Could you check a few things on this model? Use its own coordinates, in mm. A direction names the side the tool comes from. Coordinates: 2 decimals unless noted, no trailing zeros. Write each loop counter-clockwise with the first axis right and the second up, starting at its lowest first coordinate (ties: lowest second). Pieces come first, ordered by that corner, then holes.
```python
from build123d import *

# Parameters (mm, degrees)
BOSS_EXTRUDE1_DEPTH = 247.65
SKETCH2_R           = 2.286
CUT_EXTRUDE1_DEPTH  = 255.69929163
SKETCH3_R           = 2.286
CUT_EXTRUDE2_DEPTH  = 255.408366321
FILLET1_R           = 6.35


with BuildPart() as part:
    # Sketch1 → Boss-Extrude1 (new body)
    with BuildSketch(Plane.XY):
        Polygon((0, 0), (31.018857102, 0), (57.870573741, -9.773225596), (58.413530719, -8.28146356), (31.298776184, 1.5875), (0, 1.5875), align=None)
    extrude(amount=BOSS_EXTRUDE1_DEPTH)

    # Sketch2 → Cut-Extrude1 (cut, through all)
    with BuildSketch(Plane(origin=(0, 1.5875, 0), x_dir=(1, 0, 0), z_dir=(0, 1, 0))):
        with Locations(Location((4.7625, -6.35, 0), (0, 0, 180))):
            Circle(SKETCH2_R)
        with Locations(Location((4.7625, -241.3, 0), (0, 0, 180))):
            Circle(SKETCH2_R)
        with Locations(Location((4.7625, -82.55, 0), (0, 0, 180))):
            Circle(SKETCH2_R)
        with Locations(Location((4.7625, -165.1, 0), (0, 0, 180))):
            Circle(SKETCH2_R)
    extrude(amount=-CUT_EXTRUDE1_DEPTH, mode=Mode.SUBTRACT)

    # Sketch3 → Cut-Extrude2 (cut, through all)
    with BuildSketch(Plane(origin=(4.171473971, 11.461030541, 0), x_dir=(0.9396926207859064, -0.34202014332567426, 0), z_dir=(0.34202014332567426, 0.9396926207859064, 0))):
        with Locations(Location((45.023191124, -6.35, 0), (0, 0, 180))):
            Circle(SKETCH3_R)
        with Locations(Location((45.023191124, -241.3, 0), (0, 0, 180))):
            Circle(SKETCH3_R)
    extrude(amount=-CUT_EXTRUDE2_DEPTH, mode=Mode.SUBTRACT)

    # Fillet1
    fillet1_edges = [part.edges().sort_by_distance(p)[0] for p in [
        (58.14205223, -9.027344578, 0),
        (58.14205223, -9.027344578, 247.65),
    ]]
    fillet(fillet1_edges, radius=FILLET1_R)


solid = part.part
```
Item 1: I want a section at A-A, the plane z = 82.55. List the corners of the cut face in (x, y) for me, then the cut area to 3 significant figures.
Item 2: Which directions (+Z, -Z, +X, -X, +Y, -Y) give clear straight access to the entire face, cutting with the end or side of a thin tool? Please do faces 1 (the flat face through (26, 1, 247.65)), 2 (the flat face through (15, 0, 122)).
Item 3: I want a section at B-B, the plane x = 10. List the corners of the cut face in (y, z) for me.
Item 4: If I drill on line 1 along Z through (x, y) = (45, -5); line 2 along Y through (x, z) = (26, 226); line 3 along Y through (x, z) = (32, 50.5), over which ranges is the centre line in solid material (lowest first)?
Item 5: I want a section at C-C, the plane x = 41. List the corners of the cut face in (y, z) for me.
Item 6: Will these pins go through, and if not, where does the flat tip stop? pin 1 Ø7.5 at (x, z) = (4.76, 82.55) entering from -Y; pin 2 Ø4 at (x, z) = (4.76, 165.1) entering from +Y (1 decimal); pin 3 Ø12 at (x, z) = (51.5, 87) entering from -Y; pin 4 Ø7.5 at (x, z) = (4.76, 241.3) entering from +Y.
Item 7: If we mould it in two halves opening along X, with no side actions, what happens to faces 3 (the cylindrical face through (46.491, -4.775, 243.567)), 4 (the flat face through (16, 1.588, 122)), 5 (the flat face through (45, -3.4, 122.1))? For each: released by +X, released by -X, zero draft, split by the parting line, or undercut.
Taken from the geometry:
1. outline: (0, 0) - (2.48, 0) - (2.48, 1.59) - (0, 1.59) - close; (7.05, 0) - (31.02, 0) - (57.87, -9.77) - (58.41, -8.28) - (31.3, 1.59) - (7.05, 1.59) - close
1. area: 87.8 mm2
2. face 1: +Z, +X, -X, +Y, -Y
2. face 2: +Z, -Z, -X, -Y
3. outline: (0, 0) - (1.59, 0) - (1.59, 247.65) - (0, 247.65) - close
4. line 1: z = 0 to 4.31, 8.39 to 239.26, 243.34 to 247.65
4. line 2: y = 0 to 1.59
4. line 3: y = -0.36 to 1.33
5. outline: (-3.63, 0) - (-1.94, 0) - (-1.94, 247.65) - (-3.63, 247.65) - close
6. pin 1: stops at y = 0
6. pin 2: passes through
6. pin 3: stops at y = -9.64
6. pin 4: stops at y = 1.59
7. face 3: undercut
7. face 4: zero draft
7. face 5: released by +X
